Read the model definition and answer for the solid it produces. Units are mm, in the model's axes. Face numbers are marked on the shaded views. A direction names the side the tool comes from. Coordinates: 2 decimals unless noted, no trailing zeros. Loops run counter-clockwise (first coordinate to the right, second up) from the corner with the lowest first, then second, coordinate; pieces in that order, holes last. Notation, with made-up numbers: (10, -21) -> (22, -21) arc R24 cw to (22, -7) -> close; hole circle Ø1 at (83, 89.5). An arc over 180 degrees is marked (long way). Answer as CSV lines item,"result".
```python
from build123d import *

# Parameters (mm, degrees)
F0_W     = 57.15
F0_H     = 38.1
F1_DEPTH = 38.1
F2_W     = 31.75
F2_H     = 38.1
F3_DEPTH = 12.7
F5_DEPTH = 12.7
F6_W     = 31.75
F6_H     = 38.1
F7_DEPTH = 12.7
F8_DEPTH = 6.35


with BuildPart() as f1:
    # F0 (on Front) → F1 (new body)
    with BuildSketch(Plane.XZ):
        with Locations((28.575, 19.05)):
            Rectangle(F0_W, F0_H)
    extrude(amount=F1_DEPTH)

    # F2 (on face) → F3 (cut)
    with BuildSketch(Plane.XZ.offset(38.1)):
        with Locations((41.275, 19.05)):
            Rectangle(F2_W, F2_H)
        Polygon((12.7, 38.1), (25.4, 0), (25.4, 38.1), align=None)
    extrude(amount=-F3_DEPTH, mode=Mode.SUBTRACT)

    # F4 (on face) → F5 (cut)
    with BuildSketch(Plane.XZ.offset(25.4)):
        Polygon((44.45, 38.1), (57.15, 0), (57.15, 38.1), align=None)
    extrude(amount=-F5_DEPTH, mode=Mode.SUBTRACT)

    # F6 (on face) → F7 (cut)
    with BuildSketch(Plane(origin=(0, 0, 0), x_dir=(-1, 0, 0), z_dir=(0, 1, 0))):
        with Locations((-41.275, 19.05)):
            Rectangle(F6_W, F6_H)
        Polygon((-12.7, 38.1), (-25.4, 38.1), (-25.4, 0), align=None)
    extrude(amount=-F7_DEPTH, mode=Mode.SUBTRACT)

    # F8 (add): a face of the model
    f8_faces = [f1.faces().sort_by_distance(p)[0] for p in [
        (0, -19.05, 19.05),
    ]]
    extrude(f8_faces, amount=F8_DEPTH)


solid = f1.part
```
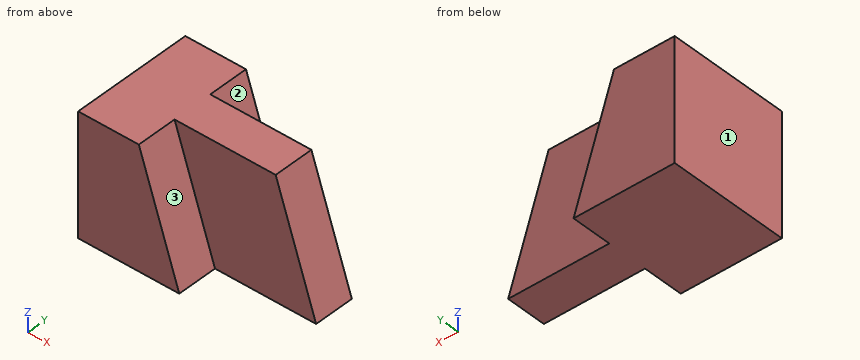
Q1. Given pin 1 Ø11.5 at (x, z) = (31.5, 18.5) entering from -Y; pin 2 Ø1 at (y, z) = (-33.5, 25.5) entering from +X, each flat-ended and moving along its own axis, determine where each tip first touches the part or whether it passes through.
Results:
pin 1,"stops at y = -25.4"
pin 2,"stops at x = 17.07"
Q2. For the marked faces 1, 2 and 3, determine the directions among +Z, -Z, +X, -X, +Y, -Y from which every point of the face is accessible in a straight line to the end or side of a thin tool.
Results:
face 1,"+Z, -Z, -X, +Y, -Y"
face 2,"+Z, +X, +Y"
face 3,"+Z, +X, -Y"
Q3. A cutting plane is placed at B-B, the plane y = -17.5. Write down the section's boundary in (x, z).
Results:
outline,"(-6.35, 0) -> (57.15, 0) -> (44.45, 38.1) -> (-6.35, 38.1) -> close"
Q4. A cutting plane is placed at C-C, the plane x = 43.5. Write down the section's boundary in (y, z).
Results:
outline,"(-25.4, 0) -> (-12.7, 0) -> (-12.7, 38.1) -> (-25.4, 38.1) -> close"
Q5. Find the intervals of material crossed by probe 1 along Y at (x, z) = (23, 22.5); probe 2 along X at (y, z) = (-25, 8); probe 3 along X at (y, z) = (-26.5, 32), in increasing order. Write a range as [from, to].
Results:
probe 1,"y = [-25.4, -12.7]"
probe 2,"x = [-6.35, 54.48]"
probe 3,"x = [-6.35, 14.73]"
Q6. A cutting plane is placed at A-A, the plane z = 33. Write down the section's boundary in (x, y).
Results:
outline,"(-6.35, -38.1) -> (14.4, -38.1) -> (14.4, -25.4) -> (46.15, -25.4) -> (46.15, -12.7) -> (14.4, -12.7) -> (14.4, 0) -> (-6.35, 0) -> close"
Q7. A cutting plane is placed at D-D, the plane z = 25. Write down the section's boundary in (x, y), and give its area (3 significant figures).
Results:
outline,"(-6.35, -38.1) -> (17.07, -38.1) -> (17.07, -25.4) -> (48.82, -25.4) -> (48.82, -12.7) -> (17.07, -12.7) -> (17.07, 0) -> (-6.35, 0) -> close"
area,"1,300 mm²"
